CAD build for the part. Positions are in the model's coordinates, mm. Coordinates: 2 decimals unless noted, no trailing zeros. Loops run counter-clockwise (first coordinate to the right, second up) from the corner with the lowest first, then second, coordinate; pieces in that order, holes last. Notation, with made-up numbers: (59.5, 84) -> (103.5, 84) arc R33 ccw to (103.5, 122) -> close; hole circle Ø1 at (11.25, -36.75). An arc over 180 degrees is marked (long way). Write item = value, one per line. Start each with the question number.
(1) Band-saw the part on D-D (y = 23). Write the cut outline in (x, z), and give its area (3 significant figures).
(2) Band-saw the part on C-C (z = 2.75). Write the cut outline in (x, y).
(3) Band-saw the part on B-B (x = 0). Write the cut outline in (y, z), and give its area (3 significant figures).
(4) Band-saw the part on A-A (y = 19.25). Write the cut outline in (x, z).
(5) Flat gauge pin, fed straight in: P1, Ø2, axis at y = 22, z = 2, coming from the -X side. Where does the tip first touch, or does it go through?
(6) Drill centre lines: line 1 (Y direction, x = 0.5, z = 1.5); line 2 (Z direction, x = 4, y = 18.75). Where is each one in solid material? Low to high. Write a range as from..to.
```python
from build123d import *

# Parameters (mm, degrees)
SKETCH2_R           = 5
BOSS_EXTRUDE1_DEPTH = 8
SKETCH4_R           = 23.702642413
SKETCH4_R_2         = 5
CUT_EXTRUDE1_DEPTH  = 28
SKETCH5_R           = 5
CUT_EXTRUDE2_DEPTH  = 18


with BuildPart() as part:
    # Sketch2 → Boss-Extrude1 (new body)
    with BuildSketch(Plane(origin=(0, 0, 0), x_dir=(1, 0, 0), z_dir=(0, 1, 0))):
        Circle(SKETCH2_R)
    extrude(amount=BOSS_EXTRUDE1_DEPTH)

    # Sketch3 one side → Revolve1 (revolve)
    with BuildSketch(Plane.XY):
        with BuildLine():
            ThreePointArc((0, 4), (7.071067812, 6.928932188), (10, 14))
            ThreePointArc((10, 14), (7.071067812, 21.071067812), (0, 24))
            Line((0, 24), (0, 4))
        make_face()
    revolve(axis=Axis((0, 24, 0), (0, -1, 0)))

    # Sketch4 → Cut-Extrude1 (cut)
    with BuildSketch(Plane.XZ):
        Circle(SKETCH4_R)
        Circle(SKETCH4_R_2, mode=Mode.SUBTRACT)
    extrude(amount=-CUT_EXTRUDE1_DEPTH, mode=Mode.SUBTRACT)

    # Sketch5 → Cut-Extrude2 (cut)
    with BuildSketch(Plane.XZ):
        Circle(SKETCH5_R)
    extrude(amount=-CUT_EXTRUDE2_DEPTH, mode=Mode.SUBTRACT)


solid = part.part
```
Findings below:
q1.outline = circle Ø8.72 at (0, 0)
q1.area = 59.7 mm²
q2.outline = (-4.18, 18) -> (4.18, 18) -> (4.18, 22.66) arc R9.61 ccw to (-4.18, 22.66) -> close
q3.outline = (18, -5) -> (22.66, -5) arc R10 ccw to (22.66, 5) -> (18, 5) -> close
q3.area = 55.7 mm²
q4.outline = circle Ø10 at (0, 0)
q5.P1 = -4.9
q6.line_1 = 18..23.87
q6.line_2 = -3..3
